from build123d import *

# Parameters (mm, degrees)
SKETCH1_R           = 5
BOSS_EXTRUDE1_DEPTH = 6
BOSS_EXTRUDE2_START = -6
SKETCH1_3_R         = 6.5
SKETCH1_3_R_2       = 5
BOSS_EXTRUDE2_DEPTH = 6
BOSS_EXTRUDE3_START = -12
SKETCH1_4_R         = 5
BOSS_EXTRUDE3_DEPTH = 12
FILLET1_R           = 1.5
SKETCH3_R           = 5.5
BOSS_EXTRUDE4_DEPTH = 2
BOSS_EXTRUDE5_START = -20
SKETCH3_2_R         = 5.5
BOSS_EXTRUDE5_DEPTH = 2
FILLET2_R           = 0.5


with BuildPart() as part:
    # Sketch1 → Boss-Extrude1 (new body)
    with BuildSketch(Plane.XY):
        Circle(SKETCH1_R)
    extrude(amount=BOSS_EXTRUDE1_DEPTH)

    # Sketch1<3> → Boss-Extrude2 (add)
    # profile 1 of 2: a face of its own
    with BuildSketch(Plane.XY.offset(BOSS_EXTRUDE2_START)):
        Circle(SKETCH1_3_R)
        Circle(SKETCH1_3_R_2, mode=Mode.SUBTRACT)
    # profile 2 of 2: a face of its own
    with BuildSketch(Plane.XY.offset(BOSS_EXTRUDE2_START)):
        Circle(SKETCH1_3_R_2)
    extrude(amount=BOSS_EXTRUDE2_DEPTH)

    # Sketch1<4> → Boss-Extrude3 (add)
    with BuildSketch(Plane.XY.offset(BOSS_EXTRUDE3_START)):
        Circle(SKETCH1_4_R)
    extrude(amount=BOSS_EXTRUDE3_DEPTH)

    # Fillet1
    fillet1_edges = [part.edges().sort_by_distance(p)[0] for p in [
        (-5, 0, -6),
        (-5, 0, 0),
    ]]
    fillet(fillet1_edges, radius=FILLET1_R - 0.0001)  # a hair under: the kernel refuses the full size

    # Sketch3 → Boss-Extrude4 (add)
    with BuildSketch(Plane.XY.offset(6)):
        Circle(SKETCH3_R)
    extrude(amount=BOSS_EXTRUDE4_DEPTH)

    # Sketch3<2> → Boss-Extrude5 (add)
    with BuildSketch(Plane.XY.offset(6).offset(BOSS_EXTRUDE5_START)):
        Circle(SKETCH3_2_R)
    extrude(amount=BOSS_EXTRUDE5_DEPTH)

    # Fillet2
    fillet2_edges = [part.edges().sort_by_distance(p)[0] for p in [
        (-5, 0, -12),
        (-5, 0, 6),
    ]]
    fillet(fillet2_edges, radius=FILLET2_R - 0.0001)  # a hair under: the kernel refuses the full size


solid = part.part
Design review of the part built by this model. Coordinates are the model's own, in mm. A direction names the side the tool comes from. Round coordinates to 2 decimals unless told otherwise and drop trailing zeros. Write each loop counter-clockwise with the first axis right and the second up, starting at its lowest first coordinate (ties: lowest second). Pieces come first, ordered by that corner, then holes. Notation, with made-up numbers: M -30,-20 L -9,-20 A19 ccw -9,-7 Z; hole C -34,38.5 d4. An arc over 180 degrees is marked long. One line per item, written item: value. Start each with the question number.
1. Take a section at C-C on z = 6.25. State the section outline as (x, y) points.
2. To check wall thickness, follow probe 1 along X at (y, z) = (-0.25, 1); probe 2 along X at (y, z) = (-1, -1.75); probe 3 along Y at (x, z) = (0.75, -5.75). State the ranges of each line that lie inside material, in increasing order. Write a range as from..to.
3. Take a section at D-D on z = 0.5. State the section outline as (x, y) points.
4. For faces 1 (the face through (-1.19, -5.37, 6.99)), 2 (the face through (-1.08, -4.88, 3.47)), 3 (the face through (-5.158, -3.955, -3.042)), list the 3-axis set-ups (+Z, -Z, +X, -X, +Y, -Y) from which the entire face can be reached by the end or side of a thin tool; tool diameter is ignored.
5. Clearance check with flat-ended pins moving along their axes: P1, Ø2, axis at y = -2, z = -5, coming from the -X side; P2, Ø3, axis at x = 4.5, z = -5, coming from the +Y side. State where each tip first meets the part, or that it passes through.
6. Draft analysis for pull direction Z (two halves, no side actions). For faces 4 (the face through (-1.19, -5.37, -13.01)), 5 (the face through (0, 0, -14)), 6 (the face through (0, 0, 8)), 7 (the face through (-1.08, -4.88, -9.53)), state which applies: pulls with the +Z half, pulls with the -Z half, needs draft (parallel to the pull), parting line crosses it, or undercut.
Computed:
1. outline: C 0,0 d11
2. probe 1: x = -5.08..5.08
2. probe 2: x = -6.42..6.42
2. probe 3: y = -6.46..6.46
3. outline: C 0,0 d10.76
4. face 1: +Z
4. face 2: none
4. face 3: +Z, -Z
5. P1: stops at x = -6.42
5. P2: stops at y = 5.77
6. face 4: needs draft
6. face 5: pulls with the -Z half
6. face 6: pulls with the +Z half
6. face 7: undercut
